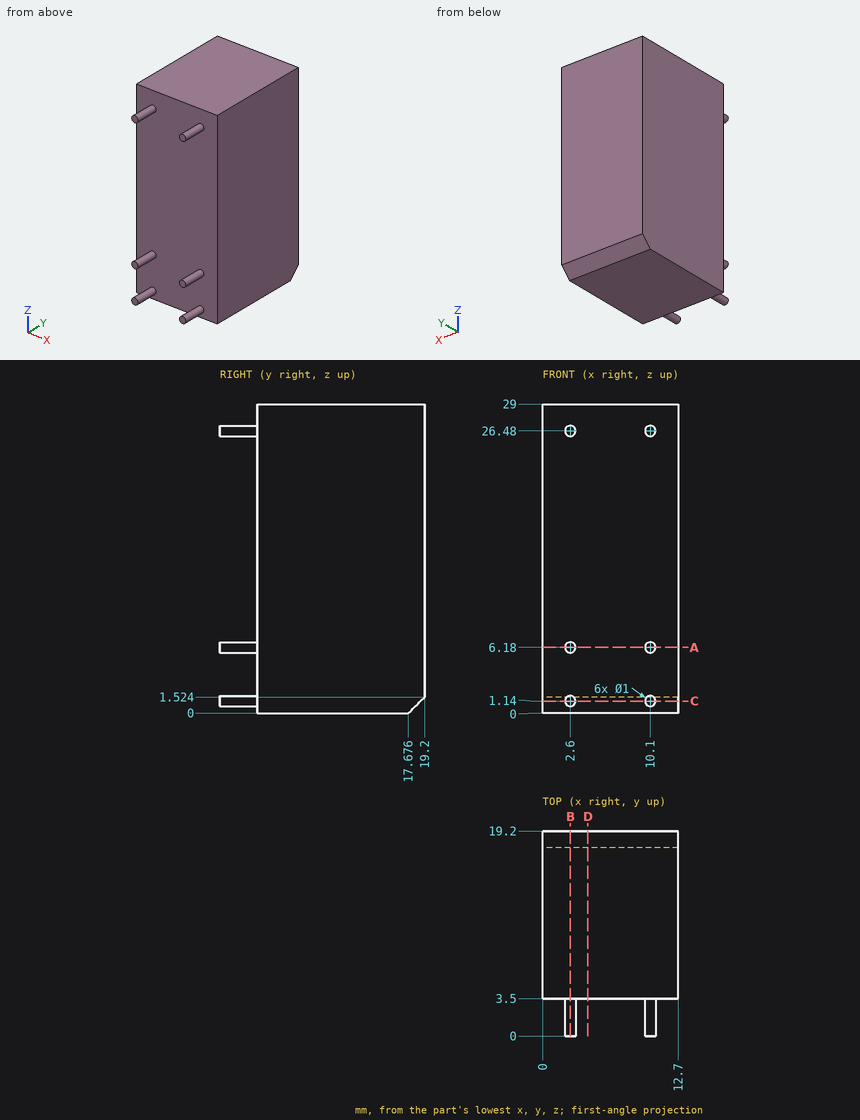
Geometry: see drawing. Coordinates: mm, zero at the bounding-box minimum. Give positions to 0.01 mm unless a question says otherwise; leave off trailing zeros. Order: outer loops, then holes, each group sorted by start corner. A loop starts at its lowest first (then second) coordinate and runs counter-clockwise, first axis right, second up. Notation, with made-up numbers: (-21.75, 52.25) -> (19.25, 52.25) arc R14 ccw to (19.25, 61.25) -> close; hole circle Ø6 at (33, 28.25). An arc over 180 degrees is marked (long way). Write item = value, one per line.
Q1. Pin query (flat end, axial travel): pin 1 (1.5 mm diameter, centred on x = 10, y = 2.5, fed in from +Z); pin 2 (4 mm diameter, centred on x = 8, z = 8.5, fed in from -Y). Return the tip coordinate at first contact, or that it passes through.
Data:
pin_1 = 26.98
pin_2 = 3.5
Q2. Cut plane A-A, the plane z = 6.18. Output: boundary loops of the cut face in (x, y), and give its area (3 significant figures).
Data:
outline = (0, 3.5) -> (2.1, 3.5) -> (2.1, 0) -> (3.1, 0) -> (3.1, 3.5) -> (9.6, 3.5) -> (9.6, 0) -> (10.6, 0) -> (10.6, 3.5) -> (12.7, 3.5) -> (12.7, 19.2) -> (0, 19.2) -> close
area = 206 mm^2
Q3. Cut plane B-B, the plane x = 2.6. Output: boundary loops of the cut face in (y, z).
Data:
outline = (0, 0.64) -> (3.5, 0.64) -> (3.5, 0) -> (17.68, 0) -> (19.2, 1.52) -> (19.2, 29) -> (3.5, 29) -> (3.5, 26.98) -> (0, 26.98) -> (0, 25.98) -> (3.5, 25.98) -> (3.5, 6.68) -> (0, 6.68) -> (0, 5.68) -> (3.5, 5.68) -> (3.5, 1.64) -> (0, 1.64) -> close
Q4. Cut plane D-D, the plane x = 4.25. Output: boundary loops of the cut face in (y, z).
Data:
outline = (3.5, 0) -> (17.68, 0) -> (19.2, 1.52) -> (19.2, 29) -> (3.5, 29) -> close
Q5. Material intervals for line 1 (Y direction, x = 6, z = 6), sorted ascending. Write a range as from..to.
Data:
line_1 = 3.5..19.2
Q6. Cut plane C-C, the plane z = 1.14. Output: boundary loops of the cut face in (x, y), and give its area (3 significant figures).
Data:
outline = (0, 3.5) -> (2.1, 3.5) -> (2.1, 0) -> (3.1, 0) -> (3.1, 3.5) -> (9.6, 3.5) -> (9.6, 0) -> (10.6, 0) -> (10.6, 3.5) -> (12.7, 3.5) -> (12.7, 18.82) -> (0, 18.82) -> close
area = 202 mm^2
